Could you check a few things on this model? Use its own coordinates, in mm. Face numbers are marked on the shaded views. Coordinates: 2 decimals unless noted, no trailing zeros. Write each loop counter-clockwise with the first axis right and the second up, starting at its lowest first coordinate (ties: lowest second). Pieces come first, ordered by that corner, then holes. Notation, with made-up numbers: M 82,33 L 96,33 A17 ccw 96,49 Z; hole C 18,-23.5 d6. An arc over 180 degrees is marked long. Answer as CSV lines item,"result". Start each with the question number.
Item 1: If I drill on line 1 along Z through (x, y) = (-1, 1.5); line 2 along Y through (x, z) = (2.25, -5.5); line 3 along Y through (x, z) = (-3, 12.25), over which ranges is the centre line in solid material (lowest first)? Write a range as [from, to].
Item 2: Suppose I cut it at B-B, the plane x = -4.25. Write out the boundary of the cut face in (y, z), and give its area (3 significant figures).
Item 3: Suppose I cut it at A-A, the plane y = 13.75. Write out the boundary of the cut face in (x, z).
Item 4: We'd pull the mould along Z, two halves only. Please class the marked faces 1, 2, 3 and 4: +Z half, -Z half, draft (parallel to the pull), parting line (faces both ways), or undercut.
Item 5: I'm going to push flat-ended pins straight in: P1, Ø0.7, axis at x = 2, z = -12.5, coming from the +Y side; P2, Ø0.6, axis at x = 0, y = -1, coming from the +Z side; P3, Ø2, axis at x = 3.5, z = -8, coming from the +Y side. Where does each tip first touch, or does it pass through?
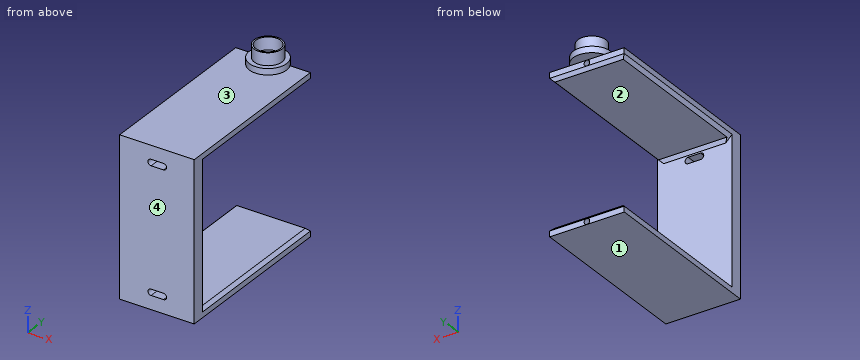
```python
from build123d import *

# Parameters (mm, degrees)
SKETCH1_W           = 12
SKETCH1_H           = 12.7
BOSS_EXTRUDE1_DEPTH = 2
SKETCH2_W           = 12
SKETCH2_H           = 1.4
BOSS_EXTRUDE2_DEPTH = 26
CHAMFER1_SIZE       = 0.5
CHAMFER2_SIZE       = 0.5
SKETCH3_R           = 0.45
CUT_EXTRUDE1_DEPTH  = 5
CUT_EXTRUDE2_DEPTH  = 5
SKETCH5_R           = 3
BOSS_EXTRUDE3_DEPTH = 1
SKETCH6_R           = 2.25
BOSS_EXTRUDE4_DEPTH = 2
SKETCH7_R           = 2
CUT_EXTRUDE3_DEPTH  = 2


with BuildPart() as part:
    # Sketch1 → Boss-Extrude1 (new body)
    with BuildSketch(Plane(origin=(0, 0, 0), x_dir=(1, 0, 0), z_dir=(0, 1, 0))):
        with Locations((0, -6.35)):
            Rectangle(SKETCH1_W, SKETCH1_H)
    boss_extrude1 = extrude(amount=-BOSS_EXTRUDE1_DEPTH)

    # Sketch2 → Boss-Extrude2 (add)
    with BuildSketch(Plane(origin=(0, 0, 0), x_dir=(1, 0, 0), z_dir=(0, 1, 0))):
        with Locations((0, -12)):
            Rectangle(SKETCH2_W, SKETCH2_H)
    boss_extrude2 = extrude(amount=BOSS_EXTRUDE2_DEPTH)

    # Mirror1: Boss-Extrude1, Boss-Extrude2 across plane
    add(boss_extrude1.mirror(Plane.XY))
    add(boss_extrude2.mirror(Plane.XY))

    # Chamfer1
    chamfer1_edges = [part.edges().sort_by_distance(p)[0] for p in [
        (-6, 13, 11.3),
        (6, 13, 11.3),
        (0, 26, 11.3),
        (0, 26, -11.3),
        (-6, 13, -11.3),
        (6, 13, -11.3),
    ]]
    chamfer(chamfer1_edges, length=CHAMFER1_SIZE)

    # Chamfer2
    chamfer2_edges = [part.edges().sort_by_distance(p)[0] for p in [
        (0, 0, -11.3),
        (0, 0, 11.3),
    ]]
    chamfer(chamfer2_edges, length=CHAMFER2_SIZE)

    # Sketch3 → Cut-Extrude1 (cut)
    with BuildSketch(Plane(origin=(0, 26, 0), x_dir=(1, 0, 0), z_dir=(0, 1, 0))):
        with Locations((0, -12.237441552)):
            Circle(SKETCH3_R)
        with Locations((0, 12.237441552)):
            Circle(SKETCH3_R)
    extrude(amount=-CUT_EXTRUDE1_DEPTH, mode=Mode.SUBTRACT)

    # Sketch4 → Cut-Extrude2 (cut)
    with BuildSketch(Plane(origin=(0, 0, 0), x_dir=(1, 0, 0), z_dir=(0, 1, 0))):
        with BuildLine():
            Line((-0.944927116, 10.523894152), (1.056095012, 10.523894152))
            ThreePointArc((1.056095012, 10.523894152), (1.556095012, 10.023894152), (1.056095012, 9.523894152))
            Line((1.056095012, 9.523894152), (-0.944927116, 9.523894152))
            ThreePointArc((-0.944927116, 9.523894152), (-1.444927116, 10.023894152), (-0.944927116, 10.523894152))
        make_face()
        with BuildLine():
            Line((-0.944927116, -10.523894152), (1.056095012, -10.523894152))
            ThreePointArc((1.056095012, -10.523894152), (1.556095012, -10.023894152), (1.056095012, -9.523894152))
            Line((1.056095012, -9.523894152), (-0.944927116, -9.523894152))
            ThreePointArc((-0.944927116, -9.523894152), (-1.444927116, -10.023894152), (-0.944927116, -10.523894152))
        make_face()
    extrude(amount=-CUT_EXTRUDE2_DEPTH, mode=Mode.SUBTRACT)

    # Sketch5 → Boss-Extrude3 (add)
    with BuildSketch(Plane.XY.offset(12.7)):
        with Locations((0, 24.785766933)):
            Circle(SKETCH5_R)
    extrude(amount=BOSS_EXTRUDE3_DEPTH)

    # Sketch6 → Boss-Extrude4 (add)
    with BuildSketch(Plane.XY.offset(13.7)):
        with Locations((0, 24.799373819)):
            Circle(SKETCH6_R)
    extrude(amount=BOSS_EXTRUDE4_DEPTH)

    # Sketch7 → Cut-Extrude3 (cut)
    with BuildSketch(Plane.XY.offset(15.7)):
        with Locations((0, 24.799373819)):
            Circle(SKETCH7_R)
    extrude(amount=-CUT_EXTRUDE3_DEPTH, mode=Mode.SUBTRACT)


solid = part.part
```
Ans:
1,line 1,"z = [-12.7, -11.3], [11.3, 12.7]"
1,line 2,"y = [-2, 0]"
1,line 3,"y = [-2, 26]"
2,outline,"M -2,-12.7 L 26,-12.7 L 26,-11.8 L 25.5,-11.3 L 0.5,-11.3 L 0,-10.8 L 0,10.8 L 0.5,11.3 L 25.5,11.3 L 26,11.8 L 26,12.7 L -2,12.7 Z"
2,area,"124 mm^2"
3,outline,"M -6,-12.7 L 6,-12.7 L 6,-11.8 L 5.5,-11.3 L -5.5,-11.3 L -6,-11.8 Z; M -6,11.8 L -5.5,11.3 L 5.5,11.3 L 6,11.8 L 6,12.7 L -6,12.7 Z"
4,face 1,"-Z half"
4,face 2,"undercut"
4,face 3,"+Z half"
4,face 4,"draft"
5,P1,"stops at y = 26"
5,P2,"stops at z = 12.7"
5,P3,"stops at y = 0"
